The listing builds one solid part. Answer for the finished solid, in the listing's coordinates (mm). A direction names the side the tool comes from. Give positions to 0.01 mm unless a question says otherwise; leave off trailing zeros. Loops run counter-clockwise (first coordinate to the right, second up) from the corner with the lowest first, then second, coordinate; pieces in that order, holes last. Notation, with made-up numbers: M 45,-30.5 L 68,-30.5 A24 ccw 68,-5.5 Z; hole C 11.5,64 d7. An arc over 180 degrees is marked long. Return JSON: item names as keys, results as strings.
from build123d import *

# Parameters (mm, degrees)
SKETCH2_W           = 50.8
SKETCH2_H           = 50.8
BOSS_EXTRUDE1_DEPTH = 1930.4
SKETCH4_W           = 38.1
SKETCH4_H           = 38.1
CUT_EXTRUDE1_DEPTH  = 2004.17710002
CUT_EXTRUDE2_DEPTH  = 1990.147718313


with BuildPart() as part:
    # Sketch2 → Boss-Extrude1 (new body)
    with BuildSketch(Plane(origin=(0, 0, 0), x_dir=(0, 0, -1), z_dir=(1, 0, 0))):
        with Locations((216.654722693, 451.762283996)):
            Rectangle(SKETCH2_W, SKETCH2_H)
    extrude(amount=BOSS_EXTRUDE1_DEPTH)

    # Sketch4 → Cut-Extrude1 (cut, through all)
    with BuildSketch(Plane.ZY):
        with Locations((-216.654722693, 451.762283996)):
            Rectangle(SKETCH4_W, SKETCH4_H)
    extrude(amount=-CUT_EXTRUDE1_DEPTH, mode=Mode.SUBTRACT)

    # Sketch5 → Cut-Extrude2 (cut, through all)
    with BuildSketch(Plane.XY.offset(-191.254722693)):
        Polygon((0, 477.162283996), (34.265032656, 426.362283996), (0, 426.362283996), align=None)
        Polygon((1164.241563896, 477.162283996), (1930.4, -658.714309068), (1930.4, 477.162283996), align=None)
    extrude(amount=-CUT_EXTRUDE2_DEPTH, mode=Mode.SUBTRACT)


solid = part.part
(1) Determine the mould class of faces 1 (the flat face through (608, 426.362, -216)), 2 (the flat face through (591, 451, -235.705)), 3 (the flat face through (591, 451, -242.055)) for opening direction Y: released by +Y, released by -Y, zero draft, split by the parting line, or undercut.
Values follow:
{"face 1": "released by -Y", "face 2": "undercut", "face 3": "zero draft"}
(2) A tool of negligible diameter and unlimited length cuts with its end or side. For faces 4 (the flat face through (16.89, 452.12, -238.88)), 5 (the flat face through (591, 451, -197.605)), from which of +Z, -Z, +X, -X, +Y, -Y can it reach the whole face along a straight path? Write none if from no direction.
Values follow:
{"face 4": "+Z, -Z, -X, -Y", "face 5": "+X, -X"}
(3) The part is cut by section A-A (z = -213.5). Determine the outline of the cut face in (x, y).
Values follow:
{"outline": "M 0,477.16 L 4.28,470.81 L 1168.52,470.81 L 1164.24,477.16 Z; M 29.98,432.71 L 34.27,426.36 L 1198.51,426.36 L 1194.22,432.71 Z"}
(4) Straight lines are drawn through the part: line 1 along Y through (x, z) = (1084, -208.5); line 2 along Z through (x, y) = (1081, 433); line 3 along X through (y, z) = (466, -194.5). For each, find the intervals that lie inside material, in ascending order.
Values follow:
{"line 1": "426.36 to 432.71, 470.81 to 477.16", "line 2": "-242.05 to -235.7, -197.6 to -191.25", "line 3": "7.53 to 1171.77"}
(5) Given pin 1 (1.5 mm diameter, centred on y = 434.5, z = -222.5, fed in from -X), flat-ended and moving along its own axis, determine where the tip first touches the part or whether it passes through.
Values follow:
{"pin 1": "through"}
(6) The part is cut by section B-B (x = 501). Determine the outline of the cut face in (y, z), and give its area (3 significant figures).
Values follow:
{"outline": "M 426.36,-242.05 L 477.16,-242.05 L 477.16,-191.25 L 426.36,-191.25 Z; hole M 432.71,-235.7 L 470.81,-235.7 L 470.81,-197.6 L 432.71,-197.6 Z", "area": "1,130 mm²"}
